Geometry: final body of the model. Coordinates: model frame, mm. Face numbers are marked on the shaded views. A direction names the side the tool comes from. Coordinates: 2 decimals unless noted, no trailing zeros. Write each loop counter-clockwise with the first axis right and the second up, starting at its lowest first coordinate (ties: lowest second). Pieces come first, ordered by that corner, then holes. Notation, with made-up numbers: M 64,3 L 116,3 A27 ccw 116,42 Z; hole C -14.75,-15.5 d6. An arc over 180 degrees is marked long. Write item = value, one per line. Start each with the question number.
Item 1: Reachability of the marked faces 4, 5 and 6 from +Z, -Z, +X, -X, +Y, -Y: full face, straight path, thin tool, end or side. Return the list, or none.
Item 2: Section C-C on x = -28. Output: boundary loops of the cut face in (y, z).
Item 3: Section D-D on z = 74.5. Output: boundary loops of the cut face in (x, y).
Item 4: Section A-A on y = -2. Output: boundary loops of the cut face in (x, z).
Item 5: Pull-direction query (Z, two-part tool) for the marked faces 1, 2 and 3; classes: +Z half, -Z half, draft (parallel to the pull), parting line (faces both ways), or undercut.
Item 6: Ray query, L1, parallel to Z at x = 11.5, y = -13; L2, parallel to X at y = -3, z = 10; L3, parallel to Y at x = -46.5, z = 34.5. Return the intervals inside material, ascending. Write a range as [from, to].
Item 7: Section B-B on x = -64. Output: boundary loops of the cut face in (y, z).
Item 8: First-contact query: pin 1 Ø16 at (y, z) = (-3.5, 35) entering from +X; pin 2 Ø2 at (x, z) = (-29.5, 70) entering from -Y; pin 3 Ø6 at (y, z) = (3, 21) entering from -X. Flat tips, straight axial feed; report the tip coordinate or a pass-through.
from build123d import *

# Parameters (mm, degrees)
SKETCH1_W           = 150
SKETCH1_H           = 20
BOSS_EXTRUDE1_DEPTH = 90
SKETCH2_W           = 162
SKETCH2_H           = 32
BOSS_EXTRUDE2_DEPTH = 5
FILLET1_R           = 10
FILLET2_R           = 10
FILLET3_R           = 10
FILLET4_R           = 10
BOSS_EXTRUDE3_DEPTH = 5
CUT_EXTRUDE1_DEPTH  = 3.5
CUT_EXTRUDE2_DEPTH  = 8


with BuildPart() as part:
    # Sketch1 → Boss-Extrude1 (new body)
    with BuildSketch(Plane.XY):
        Rectangle(SKETCH1_W, SKETCH1_H)
    extrude(amount=BOSS_EXTRUDE1_DEPTH)

    # Sketch2 → Boss-Extrude2 (add)
    with BuildSketch(Plane(origin=(0, 0, 0), x_dir=(-1, 0, 0), z_dir=(0, 0, -1))):
        Rectangle(SKETCH2_W, SKETCH2_H)
    extrude(amount=BOSS_EXTRUDE2_DEPTH)

    # Fillet1
    fillet1_edges = [part.edges().sort_by_distance(p)[0] for p in [
        (81, 16, -2.5),
    ]]
    fillet(fillet1_edges, radius=FILLET1_R)

    # Fillet2
    fillet2_edges = [part.edges().sort_by_distance(p)[0] for p in [
        (81, -16, -2.5),
    ]]
    fillet(fillet2_edges, radius=FILLET2_R)

    # Fillet3
    fillet3_edges = [part.edges().sort_by_distance(p)[0] for p in [
        (-81, 16, -2.5),
    ]]
    fillet(fillet3_edges, radius=FILLET3_R)

    # Fillet4
    fillet4_edges = [part.edges().sort_by_distance(p)[0] for p in [
        (-81, -16, -2.5),
    ]]
    fillet(fillet4_edges, radius=FILLET4_R)

    # Sketch3 → Boss-Extrude3 (add)
    with BuildSketch(Plane.XY.offset(90)):
        with BuildLine():
            Line((-81, 6), (-81, -6))
            ThreePointArc((-81, -6), (-78.071067812, -13.071067812), (-71, -16))
            Line((-71, -16), (71, -16))
            ThreePointArc((71, -16), (78.071067812, -13.071067812), (81, -6))
            Line((81, -6), (81, 6))
            ThreePointArc((81, 6), (78.071067812, 13.071067812), (71, 16))
            Line((71, 16), (-71, 16))
            ThreePointArc((-71, 16), (-78.071067812, 13.071067812), (-81, 6))
        make_face()
    extrude(amount=BOSS_EXTRUDE3_DEPTH)

    # Sketch4 → Cut-Extrude1 (cut)
    with BuildSketch(Plane.XY.offset(95)):
        with BuildLine():
            Line((-70, -11), (-45, -11))
            ThreePointArc((-45, -11), (-41.464466094, -9.535533906), (-40, -6))
            Line((-40, -6), (-40, 6))
            ThreePointArc((-40, 6), (-41.464466094, 9.535533906), (-45, 11))
            Line((-45, 11), (-70, 11))
            ThreePointArc((-70, 11), (-73.535533906, 9.535533906), (-75, 6))
            Line((-75, 6), (-75, -6))
            ThreePointArc((-75, -6), (-73.535533906, -9.535533906), (-70, -11))
        make_face()
    extrude(amount=-CUT_EXTRUDE1_DEPTH, mode=Mode.SUBTRACT)

    # Sketch5 → Cut-Extrude2 (cut)
    with BuildSketch(Plane.XY.offset(91.5)):
        with BuildLine():
            Line((-77, 6), (-77, -6))
            ThreePointArc((-77, -6), (-74.949747468, -10.949747468), (-70, -13))
            Line((-70, -13), (-45, -13))
            ThreePointArc((-45, -13), (-40.050252532, -10.949747468), (-38, -6))
            Line((-38, -6), (-38, 6))
            ThreePointArc((-38, 6), (-40.050252532, 10.949747468), (-45, 13))
            Line((-45, 13), (-70, 13))
            ThreePointArc((-70, 13), (-74.949747468, 10.949747468), (-77, 6))
        make_face()
    extrude(amount=-CUT_EXTRUDE2_DEPTH, mode=Mode.SUBTRACT)


solid = part.part
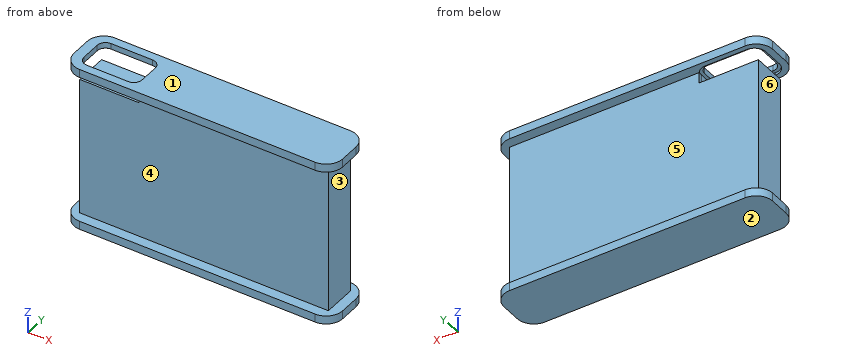
Responses:
q1.face_4 = +X, -X, -Y
q1.face_5 = +X, -X, +Y
q1.face_6 = -X, +Y, -Y
q2.outline = M -16,-5 L 16,-5 L 16,0 L 10,0 L 10,90 L 16,90 L 16,95 L -16,95 L -16,90 L -10,90 L -10,0 L -16,0 Z
q3.outline = M -75,-10 L 75,-10 L 75,10 L -75,10 Z
q4.outline = M -81,-5 L 81,-5 L 81,0 L 75,0 L 75,90 L 81,90 L 81,95 L -40,95 L -40,91.5 L -38,91.5 L -38,83.5 L -75,83.5 L -75,0 L -81,0 Z; M -81,90 L -77,90 L -77,91.5 L -75,91.5 L -75,95 L -81,95 Z
q5.face_1 = +Z half
q5.face_2 = -Z half
q5.face_3 = undercut
q6.L1 = [-5, 0], [90, 95]
q6.L2 = [-75, 75]
q6.L3 = [-10, 10]
q7.outline = M -16,-5 L 16,-5 L 16,0 L 10,0 L 10,83.5 L -10,83.5 L -10,0 L -16,0 Z; M -16,90 L -13,90 L -13,91.5 L -11,91.5 L -11,95 L -16,95 Z; M 11,91.5 L 13,91.5 L 13,90 L 16,90 L 16,95 L 11,95 Z
q8.pin_1 = 75
q8.pin_2 = -10
q8.pin_3 = -75
